from build123d import *

# Parameters (mm, degrees)
F0_W     = 30.0287567079
F0_H     = 30.0160832703
F1_DEPTH = 65.17821
F2_R     = 6.8609284015
F3_DEPTH = 24.61977
F4_SIZE  = 5.08
F6_D     = 6.35


with BuildPart() as f1:
    # F0 (on Front) → F1 (new body)
    with BuildSketch(Plane.XZ):
        with Locations((15.014378354, 15.0080416352)):
            Rectangle(F0_W, F0_H)
    extrude(amount=F1_DEPTH)

    # F2 (on face) → F3 (join)
    with BuildSketch(Plane.YZ.offset(30.0287567079)):
        with Locations((-50.9841106832, 17.3919200897)):
            Circle(F2_R)
    extrude(amount=F3_DEPTH)

    # F4
    f4_edges = [f1.edges().sort_by_distance(p)[0] for p in [
        (15.014378, 0, 30.016083),
    ]]
    chamfer(f4_edges, length=F4_SIZE)

    # F6 (through all)
    with Locations(Plane(origin=(0, 12.4680416352, 12.4680416352), x_dir=(-1, 0, 0), z_dir=(0, 0.7071067812, 0.7071067812))):
        with Locations((-14.1969984397, 21.2245760251), (-30.0287567079, 21.2245760251)):
            Hole(F6_D / 2)


solid = f1.part
Model file for the job. Use its own axes, mm. A direction names the side the tool comes from. Give positions to 0.01 mm unless a question says otherwise; leave off trailing zeros. Order: outer loops, then holes, each group sorted by start corner. A loop starts at its lowest first (then second) coordinate and runs counter-clockwise, first axis right, second up. Notation, with made-up numbers: (-28, -23) - (5, -23) arc R19 cw to (5, 1) - close; hole circle Ø4 at (73.25, -21). An arc over 180 degrees is marked (long way). Write item = value, one per line. Start each with the question number.
1. Which spindle directions (+Z, -Z, +X, -X, +Y, -Y) get a long thin tool onto all of the face, cutting with end or side? Do faces 5 (the flat face through (15, -35, 30.016)), 6 (the flat face through (30.029, -10, 10)), 7 (the cylindrical face through (42.17, -44.44, 19.45)). Say none if no direction does.
2. Cut at B-B, the plane x = 42. List the corners of the cut face in (y, z), and give its area (3 significant figures).
3. Two-plate mould, pull along Y, no slides. Class faces 1 (the flat face through (15, 0, 13)), 2 (the flat face through (0, -32, 15)), 3 (the flat face through (15, -65.178, 15)), 4 (the cylindrical face through (26.855, -17.658, 12.457)): pulls with the +Y half, pulls with the -Y half, needs draft (parallel to the pull), parting line crosses it, or undercut.
4. Probe line 1 along X through (y, z) = (-12, 6.5); line 2 along X through (y, z) = (-13.5, 18.5); line 3 along X through (y, z) = (-23, 3). List the from-to ranges inside material, lowest first.
5. Drop flat-ended pins along their axis: P1, Ø12.5, axis at y = -18.5, z = 15, coming from the +X side; P2, Ø5, axis at x = 48, z = 23, coming from the +Y side; P3, Ø1, axis at x = 44, z = 12.5, coming from the -Y side. Give the stop position or say it passes through.
6. Cut at A-A, the plane y = -55.5. List the corners of the cut face in (x, z), and give its area (3 significant figures).
Taken from the geometry:
q1.face_5 = +Z, +X, -X, +Y, -Y
q1.face_6 = +Z, -Z, +X, +Y
q1.face_7 = +X
q2.outline = circle Ø13.72 at (-50.98, 17.39)
q2.area = 148 mm²
q3.face_1 = pulls with the +Y half
q3.face_2 = needs draft
q3.face_3 = pulls with the -Y half
q3.face_4 = undercut
q4.line_1 = 0 to 30.03
q4.line_2 = 0 to 11.35, 17.05 to 27.18
q4.line_3 = 0 to 12.78, 15.62 to 28.61
q5.P1 = 30.03
q5.P2 = -44.87
q5.P3 = -56.26
q6.outline = (0, 0) - (30.03, 0) - (30.03, 12.23) - (54.65, 12.23) - (54.65, 22.56) - (30.03, 22.56) - (30.03, 30.02) - (0, 30.02) - close
q6.area = 1,160 mm²
